For this review, use the dimensioned drawing (mm, ordinates from the lowest corner) and the shaded views. A direction names the side the tool comes from. Round coordinates to 2 decimals unless told otherwise and drop trailing zeros. Write each loop counter-clockwise with the first axis right and the second up, starting at its lowest first coordinate (ties: lowest second). Pieces come first, ordered by that corner, then holes.
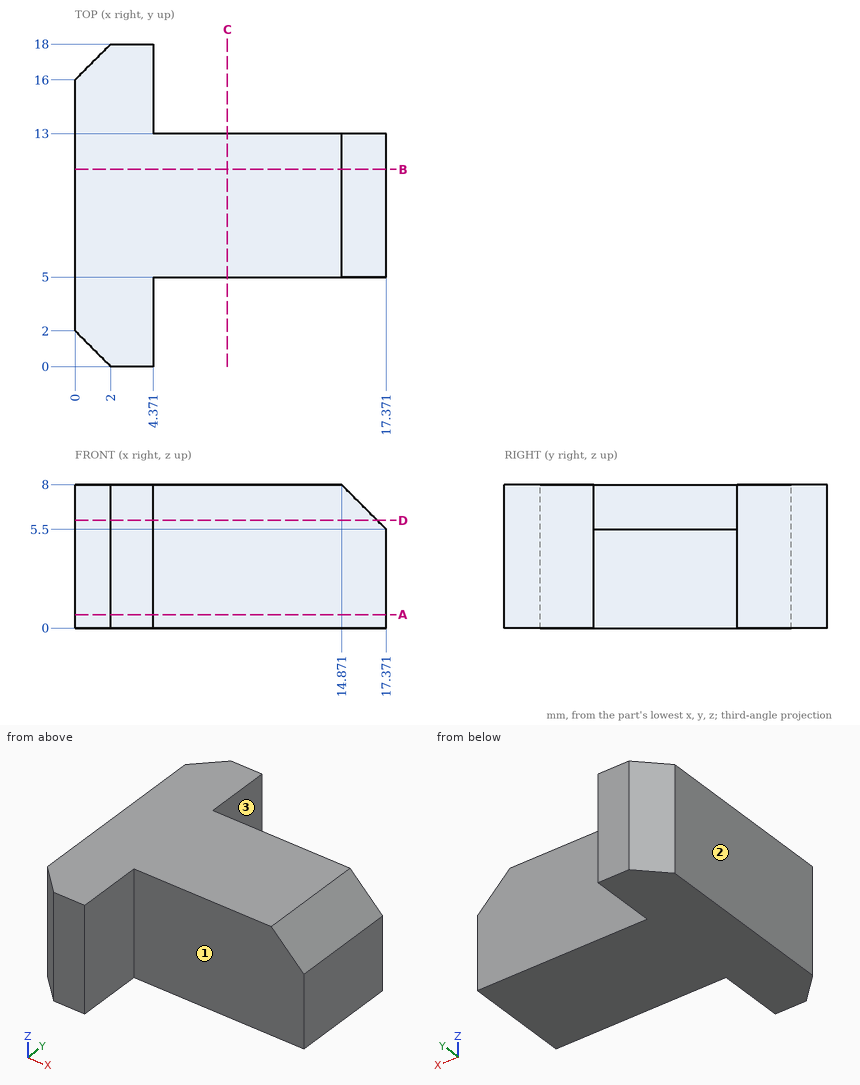
(1) We need section D-D, the plane z = 6. Give the boundary of the cut face in (x, y), and give its area (3 significant figures).
Geometry check:
outline: (0, 2) - (2, 0) - (4.37, 0) - (4.37, 5) - (16.87, 5) - (16.87, 13) - (4.37, 13) - (4.37, 18) - (2, 18) - (0, 16) - close
area: 175 mm2
(2) We need section B-B, the plane y = 11. Give the boundary of the cut face in (x, z), and give its area (3 significant figures).
Geometry check:
outline: (0, 0) - (17.37, 0) - (17.37, 5.5) - (14.87, 8) - (0, 8) - close
area: 136 mm2
(3) For line 1 along X through (y, z) = (14.75, 4.5); line 2 along Y through (x, z) = (10.5, 3.25); line 3 along X through (y, z) = (17, 2.5), list the stretches that pass through material, from the lowest coordinate up.
Geometry check:
line 1: x = 0 to 4.37
line 2: y = 5 to 13
line 3: x = 1 to 4.37
(4) We need section C-C, the plane x = 8.5. Give the boundary of the cut face in (y, z), and give its area (3 significant figures).
Geometry check:
outline: (5, 0) - (13, 0) - (13, 8) - (5, 8) - close
area: 64.0 mm2
(5) We need section A-A, the plane z = 0.75. Give the boundary of the cut face in (x, y), and give its area (3 significant figures).
Geometry check:
outline: (0, 2) - (2, 0) - (4.37, 0) - (4.37, 5) - (17.37, 5) - (17.37, 13) - (4.37, 13) - (4.37, 18) - (2, 18) - (0, 16) - close
area: 179 mm2
(6) For the marked faces 1, 2 and 3, list the 3-axis set-ups (+Z, -Z, +X, -X, +Y, -Y) from which the entire face can be reached by the end or side of a thin tool; tool diameter is ignored.
Geometry check:
face 1: +Z, -Z, +X, -Y
face 2: +Z, -Z, -X, +Y, -Y
face 3: +Z, -Z, +X, +Y
(7) For pin 1 Ø5 at (x, y) = (15.5, 11.5) entering from +Z; pin 2 Ø2.5 at (y, z) = (3, 5) entering from +X; pin 3 Ø2.5 at (x, z) = (10, 3.5) entering from -Y, all flat-tipped, find the tip position at first contact; note any pin that passes through.
Geometry check:
pin 1: stops at z = 8
pin 2: stops at x = 4.37
pin 3: stops at y = 5
